from build123d import *

# Parameters (mm, degrees)
BOSS_EXTRUDE1_DEPTH      = 30
BOSS_EXTRUDE1_DEPTH_BACK = 30
SKETCH1_W                = 150
SKETCH1_H                = 60
FILLET1_R                = 10
CHAMFER1_SIZE            = 5
CUT_EXTRUDE1_DEPTH       = 1
SKETCH14_R               = 22.5
CUT_EXTRUDE5_DEPTH       = 100


with BuildPart() as part:
    # Sketch1 → Boss-Extrude1 (new, two sides: drawn at the far end of the back side and taken through both)
    with BuildSketch(Plane.XY.offset(-BOSS_EXTRUDE1_DEPTH_BACK)):
        Rectangle(SKETCH1_W, SKETCH1_H)
    extrude(amount=BOSS_EXTRUDE1_DEPTH + BOSS_EXTRUDE1_DEPTH_BACK)

    # Fillet1
    fillet1_edges = [part.edges().sort_by_distance(p)[0] for p in [
        (0, 30, 30),
        (0, -30, 30),
        (0, -30, -30),
        (0, 30, -30),
    ]]
    fillet(fillet1_edges, radius=FILLET1_R)

    # Chamfer1
    chamfer1_edges = [part.edges().sort_by_distance(p)[0] for p in [
        (75, -30, 0),
        (75, 30, 0),
        (75, 0, 30),
        (75, 0, -30),
        (75, 27.071067812, -27.071067812),
        (75, 27.071067812, 27.071067812),
        (75, -27.071067812, 27.071067812),
        (75, -27.071067812, -27.071067812),
    ]]
    chamfer(chamfer1_edges, length=CHAMFER1_SIZE)

    # Sketch4 → Cut-Extrude1 (cut)
    # profile 1 of 2: a face of its own
    with BuildSketch(Plane.XY.offset(30)):
        with BuildLine():
            Line((34.285450061, 7.928114282), (35.631603908, 7.928114282))
            Line((35.631603908, 7.928114282), (35.631603908, -2.201092449))
            add(Edge.make_bspline(
                [(35.631603908, -2.201092449), (35.630258542, -2.388400324), (35.627675276, -2.748054301), (35.613470659, -3.266085283), (35.587184325, -3.73910251), (35.548891415, -4.168181568), (35.497804703, -4.551978234), (35.439343154, -4.893458025), (35.368574016, -5.189770949), (35.262003446, -5.522493902), (35.087257952, -5.887395922), (34.82425636, -6.281489425), (34.497544375, -6.626204042), (34.119111376, -6.925572863), (33.685649844, -7.164103854), (33.206086048, -7.335340333), (32.683372102, -7.439786861), (32.320804049, -7.450817883), (32.134007754, -7.456501103)],
                knots=[0, 0, 0, 0, 1.237770943, 2.376671248, 3.424123796, 4.367912054, 5.222547132, 5.982086412, 6.656319012, 7.234008312, 8.288027371, 9.317870876, 10.352700517, 11.413286737, 12.494591526, 13.606319346, 14.766767577, 16, 16, 16, 16], degree=3))
            add(Edge.make_bspline(
                [(32.134007754, -7.456501103), (31.988471933, -7.451869921), (31.695644221, -7.442551676), (31.259826898, -7.366601477), (30.825247001, -7.24953272), (30.389597935, -7.078093026), (29.944272615, -6.844926175), (29.483239701, -6.53984839), (29.000568882, -6.163427562), (28.682640513, -5.876122938), (28.516219292, -5.725731872)],
                knots=[0, 0, 0, 0, 0.848567217, 1.707373443, 2.573483905, 3.470863513, 4.432650262, 5.500696352, 6.691726801, 8, 8, 8, 8], degree=3))
            Line((28.516219292, -5.725731872), (29.309488523, -4.571885718))
            add(Edge.make_bspline(
                [(29.309488523, -4.571885718), (29.492500004, -4.698088845), (29.838049545, -4.936376804), (30.34592572, -5.242919377), (30.795913519, -5.505741515), (31.090269007, -5.639679854), (31.226555831, -5.701693411)],
                knots=[0, 0, 0, 0, 1.196737151, 2.259595785, 3.194191475, 4, 4, 4, 4], degree=3))
            add(Edge.make_bspline(
                [(31.226555831, -5.701693411), (31.30920288, -5.734091085), (31.471292148, -5.797630139), (31.719113918, -5.868541131), (31.96552122, -5.907294317), (32.128882765, -5.91450003), (32.209127946, -5.918039564)],
                knots=[0, 0, 0, 0, 1.051806502, 2.062826769, 3.048436908, 4, 4, 4, 4], degree=3))
            add(Edge.make_bspline(
                [(32.209127946, -5.918039564), (32.312768468, -5.913656415), (32.517627566, -5.904992544), (32.815330398, -5.82849565), (33.100150531, -5.711733923), (33.361877636, -5.540771235), (33.603100723, -5.337493718), (33.802141404, -5.091682252), (33.968072452, -4.819256606), (34.067928281, -4.561378947), (34.131548732, -4.326193389), (34.171927133, -4.110051378), (34.207235678, -3.857359327), (34.238013757, -3.567815611), (34.256032917, -3.240840545), (34.2762498, -2.877394218), (34.283558061, -2.476560309), (34.284800151, -2.197084801), (34.285450061, -2.050852064)],
                knots=[0, 0, 0, 0, 0.997221856, 1.971139923, 2.944579524, 3.951425367, 4.971190333, 5.972282193, 6.985401279, 8.033996657, 8.624075553, 9.332086008, 10.151144245, 11.082816738, 12.137127781, 13.306538797, 14.590673636, 16, 16, 16, 16], degree=3))
            Line((34.285450061, -2.050852064), (34.285450061, 7.928114282))
        make_face()
    # profile 2 of 2: a face of its own
    with BuildSketch(Plane.XY.offset(30)):
        Polygon((46.319704869, 8.312729666), (46.593142369, 8.312729666), (46.593142369, -2.071885718), (48.3239116, -2.071885718), (48.3239116, -3.610347257), (46.593142369, -3.610347257), (46.593142369, -7.071885718), (45.246988523, -7.071885718), (45.246988523, -3.610347257), (38.131603908, -3.610347257), align=None)
        Polygon((45.246988523, -2.071885718), (45.246988523, 4.442537359), (40.775834677, -2.071885718), align=None, mode=Mode.SUBTRACT)
    extrude(amount=-CUT_EXTRUDE1_DEPTH, mode=Mode.SUBTRACT)

    # Sketch14 → Cut-Extrude5 (cut)
    with BuildSketch(Plane.ZY.offset(75)):
        Circle(SKETCH14_R)
    extrude(amount=-CUT_EXTRUDE5_DEPTH, mode=Mode.SUBTRACT)


solid = part.part
Geometry check sheet. Reference: the model listing, model coordinates, mm. A direction names the side the tool comes from. Coordinates: 2 decimals unless noted, no trailing zeros. Order: outer loops, then holes, each group sorted by start corner. A loop starts at its lowest first (then second) coordinate and runs counter-clockwise, first axis right, second up. Notation, with made-up numbers: M 22,-18 L 65,-18 A27 cw 65,10 Z; hole C -9,-23.75 d5. An arc over 180 degrees is marked long. Use CSV: the item, a comma, the result in double quotes.
Item 1: Cross-section at C-C on x = 27. Record the cut outline in (y, z), then the cut area to 3 significant figures.
Returned:
outline,"M -30,-20 A10 ccw -20,-30 L 20,-30 A10 ccw 30,-20 L 30,20 A10 ccw 20,30 L -20,30 A10 ccw -30,20 Z"
area,"3,510 mm2"
Item 2: Tool access check on faces 5 (the flat face through (25, 0, 0)), 6 (the flat face through (-75, 13, 20)), 7 (the flat face through (34.5, -1.4, 29)). Record the directions out of +Z, -Z, +X, -X, +Y, -Y that give a thin tool (end or side, any length) a straight path to the whole face; none if there is none.
Returned:
face 5,"-X"
face 6,"+Z, -Z, -X, +Y, -Y"
face 7,"+Z"
Item 3: Cross-section at D-D on y = 2. Record the cut outline in (x, z), then the cut area to 3 significant figures.
Returned:
outline,"M -75,-30 L 70,-30 L 75,-25 L 75,25 L 70,30 L 46.59,30 L 46.59,29 L 45.25,29 L 45.25,30 L 43.57,30 L 43.57,29 L 41.98,29 L 41.98,30 L 35.63,30 L 35.63,29 L 34.29,29 L 34.29,30 L -75,30 L -75,22.41 L 25,22.41 L 25,-22.41 L -75,-22.41 Z"
area,"4,490 mm2"
Item 4: Cross-section at B-B on z = 0. Record the cut outline in (x, y).
Returned:
outline,"M -75,-30 L 70,-30 L 75,-25 L 75,25 L 70,30 L -75,30 L -75,22.5 L 25,22.5 L 25,-22.5 L -75,-22.5 Z"
Item 5: Mould release check, pull along Y, two halves, no side actions. Record for faces 1 (the conical face through (73.09, -24.83, -24.94)), 2 (the cylindrical face through (-25.7, -19.961, 10.382)), 3 (the flat face through (-4, 0, 30)), 4 (the flat face through (43.04, 1.23, 29.51)): pulls with the +Y half, pulls with the -Y half, needs draft (parallel to the pull), parting line crosses it, or undercut.
Returned:
face 1,"pulls with the -Y half"
face 2,"undercut"
face 3,"needs draft"
face 4,"undercut"
Item 6: Thickness scan on line 1 along Y through (x, z) = (-23, 0); line 2 along X through (y, z) = (19.5, 2.5); line 3 along Z through (x, y) = (-66, 7). Record the ranges inside material, lowest first.
Returned:
line 1,"y = -30 to -22.5, 22.5 to 30"
line 2,"x = 25 to 75"
line 3,"z = -30 to -21.38, 21.38 to 30"
Item 7: Gauge pin test, flat ends, axial feed: pin 1 Ø0.8 at (x, z) = (47, 29.5) entering from +Y; pin 2 Ø22.5 at (y, z) = (7, 1.5) entering from -X; pin 3 Ø0.5 at (y, z) = (3, 29.5) entering from +X. Record the tip position at first contact, or that the pin passes through.
Returned:
pin 1,"stops at y = 24.15"
pin 2,"stops at x = 25"
pin 3,"stops at x = 70.75"
Item 8: Cross-section at A-A on x = -5.5. Record the cut outline in (y, z).
Returned:
outline,"M -30,-20 A10 ccw -20,-30 L 20,-30 A10 ccw 30,-20 L 30,20 A10 ccw 20,30 L -20,30 A10 ccw -30,20 Z; hole C 0,0 d45"
